```python
from build123d import *

# Parameters (mm, degrees)
F0_W     = 76.2
F0_H     = 76.2
F0_R     = 3.175
F1_DEPTH = 3.175
F2_SIZE  = 3.17499


# Not quite as in the source:
# - a fillet or chamfer is up to 0.001 mm smaller than in the source, because OpenCascade refuses the exact size


with BuildPart() as f1:
    # F0 (on Top) → F1 (new body)
    with BuildSketch(Plane.XY):
        with Locations((38.1, 38.1)):
            Rectangle(F0_W, F0_H)
        with Locations((38.1, 15.875)):
            Circle(F0_R, mode=Mode.SUBTRACT)
    extrude(amount=F1_DEPTH)

    # F2 (size 3.175 in the source; OpenCascade refuses exactly that, so slightly less here)
    f2_edges = [f1.edges().sort_by_distance(p)[0] for p in [
        (38.1, 76.2, 3.175),
        (76.2, 38.1, 3.175),
        (38.1, 0, 3.175),
        (0, 38.1, 3.175),
    ]]
    chamfer(f2_edges, length=F2_SIZE)


solid = f1.part
```
CAD build for the part. Positions are in the model's coordinates, mm. Give positions to 0.01 mm unless a question says otherwise; leave off trailing zeros. Order: outer loops, then holes, each group sorted by start corner. A loop starts at its lowest first (then second) coordinate and runs counter-clockwise, first axis right, second up.
(1) Drill centre lines: L1, parallel to Y at x = 40, z = 0.7; L2, parallel to Y at x = 8.5, z = 2.05; L3, parallel to X at y = 66, z = 1.3. Where is each one in solid material? Low to high.
(2) Saw through at D-D, the plane z = 2. Give the cut face in (x, y) (3 decimals), then the cut area to 3 significant figures.
(3) Mould opens along Y. For faces 1 (the cylindrical face through (34.928, 16.015, 1.565)), 2 (the flat face through (2, 38, 2)), 3 (the flat face through (37.6, 74.6, 1.6)) say: released by +Y, released by -Y, zero draft, split by the parting line, or undercut.
(4) Flat gauge pin, fed straight in: pin 1 (1 mm diameter, centred on y = 28.5, z = 2.5, fed in from +X). Where does the tip first touch, or does it go through?
Results found:
1. L1: y = 0.7 to 13.33, 18.42 to 75.5
1. L2: y = 2.05 to 74.15
1. L3: x = 1.3 to 74.9
2. outline: (2, 2) - (74.2, 2) - (74.2, 74.2) - (2, 74.2) - close; hole circle Ø6.35 at (38.1, 15.875)
2. area: 5,180 mm2
3. face 1: undercut
3. face 2: zero draft
3. face 3: released by +Y
4. pin 1: stops at x = 74.2
